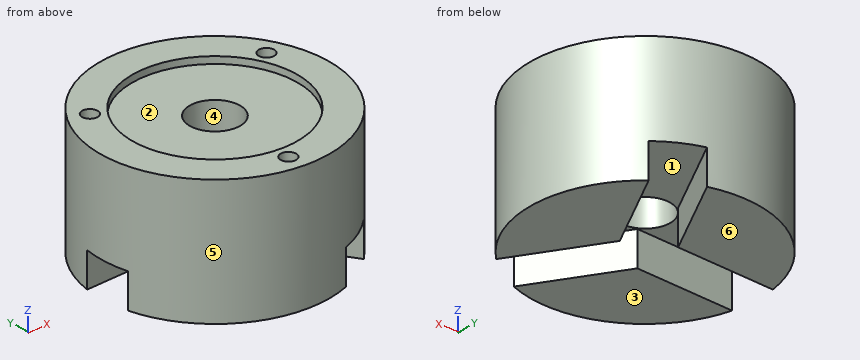
from build123d import *

# Parameters (mm, degrees)
SKETCH1_R                  = 50
BOSS_EXTRUDE1_DEPTH        = 55
SKETCH2_R                  = 36
CUT_EXTRUDE1_DEPTH         = 3
CUT_EXTRUDE2_REACH         = 89.772
SKETCH3_R                  = 11
M8X1_25_TAPPED_HOLE1_D     = 6.8
M8X1_25_TAPPED_HOLE1_DEPTH = 10.25
M8X1_25_TAPPED_HOLE1_TIP   = 2.042926105
CUT_EXTRUDE3_DEPTH         = 15


with BuildPart() as part:
    # Sketch1 → Boss-Extrude1 (new body)
    with BuildSketch(Plane.XY):
        Circle(SKETCH1_R)
    extrude(amount=BOSS_EXTRUDE1_DEPTH)

    # Sketch2 → Cut-Extrude1 (cut)
    with BuildSketch(Plane.XY.offset(55)):
        Circle(SKETCH2_R)
    extrude(amount=-CUT_EXTRUDE1_DEPTH, mode=Mode.SUBTRACT)

    # Sketch3 → Cut-Extrude2 (cut, up to next)
    with BuildSketch(Plane.XY.offset(52), mode=Mode.PRIVATE) as cut_extrude2_sk1:
        Circle(SKETCH3_R)
    cut_extrude2_tool1 = extrude(cut_extrude2_sk1.sketch, amount=-CUT_EXTRUDE2_REACH, mode=Mode.PRIVATE) & part.part
    add(cut_extrude2_tool1.solids().sort_by_distance((0, 0, 52))[0], mode=Mode.SUBTRACT)

    # M8x1.25 Tapped Hole1
    with Locations(Plane.XY.offset(55)):
        with Locations((-34.068677595, 24.562679147), (38.306242924, 17.223000697), (-4.237565329, -41.785679845), (0, 0)):
            Hole(M8X1_25_TAPPED_HOLE1_D / 2, depth=M8X1_25_TAPPED_HOLE1_DEPTH)
            with Locations((0, 0, -(M8X1_25_TAPPED_HOLE1_DEPTH + M8X1_25_TAPPED_HOLE1_TIP / 2))):  # 118° drill point
                Cone(0, M8X1_25_TAPPED_HOLE1_D / 2, M8X1_25_TAPPED_HOLE1_TIP, mode=Mode.SUBTRACT)

    # Sketch7 → Cut-Extrude3 (cut)
    with BuildSketch(Plane(origin=(0, 0, 0), x_dir=(-1, 0, 0), z_dir=(0, 0, -1))):
        Polygon((-56.730768418, 82.955529741), (-11.543830818, 0.270745983), (-60.557485259, -80.204681778), (-43.476211931, -90.608051497), (5.53744251, -10.132623736), (99.738034552, -12.341979735), (100.20698035, 7.652521756), (6.006388308, 9.861877754), (-39.180549293, 92.546661513), align=None)
    extrude(amount=-CUT_EXTRUDE3_DEPTH, mode=Mode.SUBTRACT)


solid = part.part
Part model, mm, in its own coordinate system. Face numbers are marked on the shaded views. A direction names the side the tool comes from. Round coordinates to 2 decimals unless told otherwise and drop trailing zeros. Write each loop counter-clockwise with the first axis right and the second up, starting at its lowest first coordinate (ties: lowest second). Pieces come first, ordered by that corner, then holes. Notation, with made-up numbers: M -14,39 L 16,39 A32 ccw 16,74 Z; hole C 2,74.5 d3. An arc over 180 degrees is marked long. Return JSON: item names as keys, results as strings. Group by question number.
(1) Pin check, flat tips, straight feed: pin 1 Ø1 at (x, z) = (-14, 7) entering from -Y; pin 2 Ø2 at (x, z) = (11, 48) entering from +Y; pin 3 Ø5 at (x, z) = (29.5, 8.5) entering from -Y. Stop position of each tip, or through.
(2) Which spindle directions (+Z, -Z, +X, -X, +Y, -Y) get a long thin tool onto all of the face, cutting with end or side? Do the marked faces 1, 2 and 3. Say none if no direction does.
(3) Saw through at A-A on z = 11. Write the cut outline in (x, y).
(4) Two-plate mould, pull along Y, no slides. Class the marked faces 4, 5 and 6: +Y half, -Y half, draft (parallel to the pull), parting line (faces both ways), or undercut.
(5) Saw through at D-D on x = -40.5. Write the cut outline in (y, z).
(6) Saw through at C-C on x = -24.5. Write the cut outline in (y, z), then the cut area to 3 significant figures.
(7) Saw through at B-B on z = 22.5. Write the cut outline in (x, y).
(8) Drill centre lines: probe 1 along Y at (x, z) = (0, 30); probe 2 along X at (y, z) = (-6, 43.5); probe 3 along Z at (x, y) = (-29, -15.5). Where is each one in solid material? Low to high.
Returned:
{
 "1": {"pin 1": "y = -48.14", "pin 2": "y = 48.99", "pin 3": "y = -33.32"},
 "2": {"face 1": "-Z", "face 2": "+Z", "face 3": "-Z, +X, -X, +Y, -Y"},
 "3": {"outline": "M -49.21,8.85 L -6.01,9.86 L 14.72,47.78 A50 ccw Z; M -48.74,-11.15 A50 ccw 16.94,-47.04 L -5.54,-10.13 Z; M 11.54,0.27 L 34.02,-36.64 A50 ccw 32.27,38.19 Z"},
 "4": {"face 4": "undercut", "face 5": "parting line", "face 6": "draft"},
 "5": {"outline": "M -29.32,0 L -10.95,0 L -10.95,15 L 9.05,15 L 9.05,0 L 29.32,0 L 29.32,55 L -29.32,55 Z"},
 "6": {"outline": "M -43.59,0 L -10.58,0 L -10.58,15 L 9.43,15 L 9.43,0 L 43.59,0 L 43.59,55 L 26.38,55 L 26.38,52 L -26.38,52 L -26.38,55 L -43.59,55 Z", "area": "4,340 mm²"},
 "7": {"outline": "C 0,0 d100; hole C 0,0 d22"},
 "8": {"probe 1": "-50 to -11, 11 to 50", "probe 2": "-49.64 to -9.22, 9.22 to 49.64", "probe 3": "0 to 52"}
}
